from build123d import *

# Parameters (mm, degrees)
F0_R     = 11
F1_DEPTH = 1.8
F2_R     = 3.95
F3_DEPTH = 5.5
F4_R     = 5
F5_DEPTH = 2.5


with BuildPart() as f1:
    # F0 (on Front) → F1 (new body)
    with BuildSketch(Plane.XZ):
        Circle(F0_R)
    extrude(amount=F1_DEPTH)

    # F2 (on Front) → F3 (join)
    with BuildSketch(Plane.XZ):
        Circle(F2_R)
    extrude(amount=F3_DEPTH)

    # F4 (on Front) → F5 (join)
    with BuildSketch(Plane.XZ):
        Circle(F4_R)
    extrude(amount=F5_DEPTH)


solid = f1.part
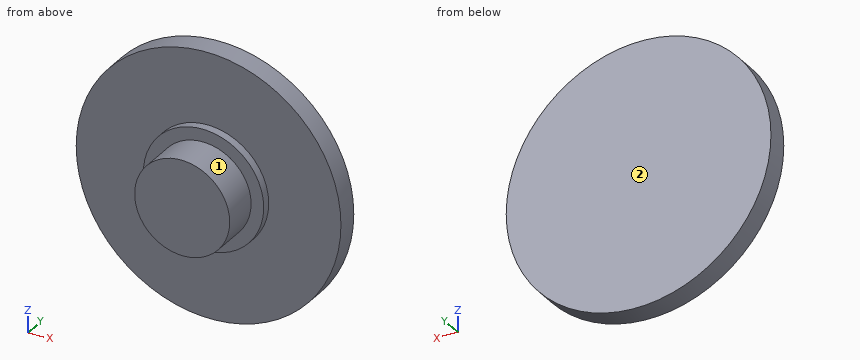
Here's how the part is built. I have some questions about the finished solid (model axes, mm). Face numbers are marked on the shaded views. A direction names the side the tool comes from. Coordinates: 2 decimals unless noted, no trailing zeros. Loops run counter-clockwise (first coordinate to the right, second up) from the corner with the lowest first, then second, coordinate; pieces in that order, holes last.
1. Imagine slicing it at B-B, the plane x = 3.5. Please give me the cut outline in (y, z).
2. I need wall thicknesses on L1, parallel to Y at x = -7, z = -2.25; L2, parallel to X at y = -4.45, z = -1.25; L3, parallel to X at y = -2.6, z = 3. Which ranges of each line are inside material? Lowest first, please.
3. For the marked faces 1 and 2, which set-ups out of +Z, -Z, +X, -X, +Y, -Y let a thin tool reach every point of the face, with its end or its side?
4. Imagine slicing it at A-A, the plane z = 0. Please give me the cut outline in (x, y).
5. For P1, Ø3, axis at y = -1.5, z = -2, coming from the +X side; P2, Ø3, axis at x = -3.5, z = -6.5, coming from the -Y side; P3, Ø1, axis at x = -4, y = -1.5, coming from the -Z side, each with a flat end and sliding along its axis, tell me the tip position at first contact or that it passes through.
6. Imagine slicing it at C-C, the plane y = -4.4. Please give me the cut outline in (x, z), and give its area (3 significant figures).
7. Imagine slicing it at D-D, the plane y = -1.3. Please give me the cut outline in (x, z), and give its area (3 significant figures).
Taken from the geometry:
1. outline: (-5.5, -1.83) - (-2.5, -1.83) - (-2.5, -3.57) - (-1.8, -3.57) - (-1.8, -10.43) - (0, -10.43) - (0, 10.43) - (-1.8, 10.43) - (-1.8, 3.57) - (-2.5, 3.57) - (-2.5, 1.83) - (-5.5, 1.83) - close
2. L1: y = -1.8 to 0
2. L2: x = -3.75 to 3.75
2. L3: x = -2.57 to 2.57
3. face 1: -Y
3. face 2: +Z, -Z, +X, -X, +Y
4. outline: (-11, -1.8) - (-5, -1.8) - (-5, -2.5) - (-3.95, -2.5) - (-3.95, -5.5) - (3.95, -5.5) - (3.95, -2.5) - (5, -2.5) - (5, -1.8) - (11, -1.8) - (11, 0) - (-11, 0) - close
5. P1: stops at x = 10.99
5. P2: stops at y = -1.8
5. P3: stops at z = -10.43
6. outline: circle Ø7.9 at (0, 0)
6. area: 49.0 mm2
7. outline: circle Ø22 at (0, 0)
7. area: 380 mm2
